```python
from build123d import *


with BuildPart() as part:
    # Sketch → Revolution (revolve)
    with BuildSketch(Plane.XZ):
        with BuildLine():
            Line((0, 5.25), (8, 5.25))
            Line((8, 5.25), (8, 3.75))
            Line((8, 3.75), (12.34, 3.75))
            Line((12.34, 3.75), (12.85, 2.24))
            Line((12.85, 2.24), (13.760654, 2.24))
            Line((13.760654, 2.24), (14, 1))
            Line((14, 1), (13.99, 0.648005))
            Line((13.99, 0.648005), (13.315, 0.65))
            Line((13.315, 0.65), (13.315, 0))
            Line((13.315, 0), (12.535, 0))
            Line((12.535, 0), (12.535, 0.8))
            Line((12.535, 0.8), (6.9, 1.137238))
            ThreePointArc((0, 0), (3.496546, 0.286211), (6.9, 1.137238))
            Line((0, 0), (0, 5.25))
        make_face()
    revolve(axis=Axis((0, 0, 0), (0, 0, 1)))


solid = part.part
```
The listing builds one solid part. Answer for the finished solid, in the listing's coordinates (mm). A direction names the side the tool comes from. Give positions to 0.01 mm unless a question says otherwise; leave off trailing zeros. Write each loop counter-clockwise with the first axis right and the second up, starting at its lowest first coordinate (ties: lowest second). Pieces come first, ordered by that corner, then holes. Notation, with made-up numbers: (1.25, 54) -> (22.25, 54) arc R19 cw to (22.25, 58) -> close; hole circle Ø10 at (-4, 21.25). An arc over 180 degrees is marked (long way). Use one line per item in the form item = value.
1) Section A-A on z = 4.45 is taken. Write down the section's boundary in (x, y), plus the area to 3 significant figures.
Result:
outline = circle Ø16 at (0, 0)
area = 201 mm²
2) For a pull along Y with two mould halves and no side action, classify faces 3 (the flat face through (0, 0, 5.25)), 4 (the conical face through (-5.69, -4.37, 1.12)), 5 (the cylindrical face through (11.956, 3.765, 0.406)), 6 (the cylindrical face through (12.7, 4, 0.3)) as +Y half, -Y half, draft (parallel to the pull), parting line (faces both ways), or undercut.
Result:
face_3 = draft
face_4 = undercut
face_5 = undercut
face_6 = parting line
3) Straight lines are drawn through the part: probe 1 along X at (y, z) = (10.75, 0.6); probe 2 along Z at (x, y) = (8.75, 3); probe 3 along X at (y, z) = (10.5, 0.6). For each, find the intervals that lie inside material, in ascending order.
Result:
probe_1 = -7.86 to -6.45, 6.45 to 7.86
probe_2 = 1 to 3.75
probe_3 = -8.19 to -6.85, 6.85 to 8.19
4) A tool of negligible diameter and unlimited length cuts with its end or side. For faces 1 (the flat face through (10, -8, 0)), 2 (the cylindrical face through (-1.73, -7.81, 4.49)), from which of +Z, -Z, +X, -X, +Y, -Y can it reach the whole face along a straight path? Write none if from no direction.
Result:
face_1 = -Z, +X, -X, +Y, -Y
face_2 = +Z
5) Each of these flat-tipped pins is pushed along its axis until it touches: P1, Ø3, axis at x = 6, y = 5, coming from the -Z side; P2, Ø1.5, axis at y = 3.5, z = 3.5, coming from the -X side; P3, Ø3, axis at y = 2, z = 4, coming from the -X side. Where does it stop, or does it pass through?
Result:
P1 = 0.95
P2 = -12.25
P3 = -12.64
6) Section B-B on z = 2.8 is taken. Write down the section's boundary in (x, y), plus the area to 3 significant figures.
Result:
outline = circle Ø25.32 at (0, 0)
area = 504 mm²
